from build123d import *

# Parameters (mm, degrees)
SKETCH2_W           = 12.7
SKETCH2_H           = 44.45
BOSS_EXTRUDE1_DEPTH = 15.88
SKETCH4_W           = 12.7
SKETCH4_H           = 25.4
BOSS_EXTRUDE2_DEPTH = 20.32
SKETCH5_R           = 6.35
CUT_EXTRUDE1_DEPTH  = 12.7
SKETCH6_R           = 2.11
CUT_EXTRUDE2_DEPTH  = 20.7
SKETCH7_R           = 2.11
CUT_EXTRUDE3_DEPTH  = 16.7


with BuildPart() as part:
    # Sketch2 → Boss-Extrude1 (new body)
    with BuildSketch(Plane(origin=(0, 0, 0), x_dir=(1, 0, 0), z_dir=(0, 1, 0))):
        with Locations((6.35, 22.225)):
            Rectangle(SKETCH2_W, SKETCH2_H)
    extrude(amount=BOSS_EXTRUDE1_DEPTH)

    # Sketch4 → Boss-Extrude2 (add)
    with BuildSketch(Plane(origin=(0, 15.88, 0), x_dir=(1, 0, 0), z_dir=(0, 1, 0))):
        with Locations((6.35, 22.23)):
            Rectangle(SKETCH4_W, SKETCH4_H)
    extrude(amount=BOSS_EXTRUDE2_DEPTH)

    # Sketch5 → Cut-Extrude1 (cut)
    with BuildSketch(Plane(origin=(12.7, 0, 0), x_dir=(0, 0, -1), z_dir=(1, 0, 0))):
        with Locations((22.23, 26.04)):
            Circle(SKETCH5_R)
    extrude(amount=-CUT_EXTRUDE1_DEPTH, mode=Mode.SUBTRACT)

    # Sketch6 → Cut-Extrude2 (cut)
    with BuildSketch(Plane(origin=(0, 15.88, 0), x_dir=(1, 0, 0), z_dir=(0, 1, 0))):
        with Locations((6.35, 39.69)):
            Circle(SKETCH6_R)
    extrude(amount=-CUT_EXTRUDE2_DEPTH, mode=Mode.SUBTRACT)

    # Sketch7 → Cut-Extrude3 (cut)
    with BuildSketch(Plane(origin=(0, 15.88, 0), x_dir=(1, 0, 0), z_dir=(0, 1, 0))):
        with Locations((6.35, 4.765)):
            Circle(SKETCH7_R)
    extrude(amount=-CUT_EXTRUDE3_DEPTH, mode=Mode.SUBTRACT)


solid = part.part
Work out the finished part from the listing and answer in its coordinate system (mm). A direction names the side the tool comes from. Round coordinates to 2 decimals unless told otherwise and drop trailing zeros. Write each loop counter-clockwise with the first axis right and the second up, starting at its lowest first coordinate (ties: lowest second). Pieces come first, ordered by that corner, then holes. Notation, with made-up numbers: M 78.25,31.25 L 83.25,31.25 A12 ccw 83.25,36.25 Z; hole C 61,51 d6. An arc over 180 degrees is marked long. Use a Markdown table: item, result.
1) The part is cut by section A-A on x = 6.35. Give the vertices of the cut face in (y, z) (3 decimals), plus the area to 3 significant figures.
Taken from the geometry:
| item | result |
|---|---|
| outline | M 0,-44.45 L 15.88,-44.45 L 15.88,-41.8 L 0,-41.8 Z; M 0,-37.58 L 15.88,-37.58 L 15.88,-34.93 L 36.2,-34.93 L 36.2,-9.53 L 15.88,-9.53 L 15.88,-6.875 L 0,-6.875 Z; M 0,-2.655 L 15.88,-2.655 L 15.88,0 L 0,0 Z; hole C 26.04,-22.23 d12.7 |
| area | 961 mm2 |
2) The part is cut by section B-B on y = 26.04. Give the vertices of the cut face in (x, z), plus the area to 3 significant figures.
Taken from the geometry:
| item | result |
|---|---|
| outline | M 0,-34.93 L 12.7,-34.93 L 12.7,-28.58 L 0,-28.58 Z; M 0,-15.88 L 12.7,-15.88 L 12.7,-9.53 L 0,-9.53 Z |
| area | 161 mm2 |
3) The part is cut by section D-D on x = 10. Give the vertices of the cut face in (y, z), plus the area to 3 significant figures.
Taken from the geometry:
| item | result |
|---|---|
| outline | M 0,-44.45 L 15.88,-44.45 L 15.88,-34.93 L 36.2,-34.93 L 36.2,-9.53 L 15.88,-9.53 L 15.88,0 L 0,0 Z; hole C 26.04,-22.23 d12.7 |
| area | 1,100 mm2 |
4) The part is cut by section C-C on z = -39.69. Give the vertices of the cut face in (x, y).
Taken from the geometry:
| item | result |
|---|---|
| outline | M 0,0 L 4.24,0 L 4.24,15.88 L 0,15.88 Z; M 8.46,0 L 12.7,0 L 12.7,15.88 L 8.46,15.88 Z |
5) Flat-ended cylindrical pins translate along their axes: pin 1 (2.5 mm diameter, centred on x = 6.35, z = -39.69, fed in from +Y); pin 2 (1 mm diameter, centred on x = 10, y = 25, fed in from -Z); pin 3 (7.5 mm diameter, centred on x = 6.5, z = -3.5, fed in from +Y). Find the tip coordinate at first contact, or state that the pin passes through.
Taken from the geometry:
| item | result |
|---|---|
| pin 1 | passes through |
| pin 2 | stops at z = -34.93 |
| pin 3 | stops at y = 15.88 |
6) Determine the mould class of faces 4 (the face through (4.242, 8.051, -4.858)), 5 (the face through (6, 8, 0)), 6 (the face through (6, 0, -23)) for opening direction Z: pulls with the +Z half, pulls with the -Z half, needs draft (parallel to the pull), parting line crosses it, or undercut.
Taken from the geometry:
| item | result |
|---|---|
| face 4 | undercut |
| face 5 | pulls with the +Z half |
| face 6 | needs draft |
7) Consider line 1 (Z direction, x = 6.35, y = 8.5) (3 decimals); line 2 (Y direction, x = 6.75, z = -22.23); line 3 (Z direction, x = 7.25, y = 12). Determine where each line is inside the solid, lowest interval first. Write a range as [from, to].
Taken from the geometry:
| item | result |
|---|---|
| line 1 | z = [-44.45, -41.8], [-37.58, -6.875], [-2.655, 0] |
| line 2 | y = [0, 19.69], [32.39, 36.2] |
| line 3 | z = [-44.45, -41.6], [-37.78, -6.67], [-2.86, 0] |
8) Which of the six approach directions +Z, -Z, +X, -X, +Y, -Y give full straight-line access (tool end or side, diameter ignored) to faces 1 (the face through (6, 15.88, -7)), 2 (the face through (6, 15.88, -42)), 3 (the face through (5.89, 8.05, -37.63))?
Taken from the geometry:
| item | result |
|---|---|
| face 1 | +Z, +X, -X, +Y |
| face 2 | -Z, +X, -X, +Y |
| face 3 | +Y, -Y |
